Autodesk Fusion 360 part; units mm, degrees
sketch "Sketch1" plane through (0, 0, 0) normal (0, 1, 0) x (1, 0, 0)
  line L0 (0, 0) -> (20, 0)
  line L1 (20, 0) -> (20, 13)
  line L2 (20, 13) -> (0, 13)
  line L3 (0, 3) -> (11, 3)
  line L4 (11, 3) -> (11, 10)
  line L5 (11, 10) -> (0, 10)
  line L6 (0, 13) -> (0, 10)
  line L7 (0, 3) -> (0, 0)
  circle A0 centre (15.5354, 6.5333) radius 3
  dimension "d2" = 6
sketch "Sketch2" plane through (0, 0, 0) normal (0, 1, 0) x (-1, 0, 0)
  line L0 (0, -3) -> (-11, -3)
  line L1 (-20, -13) -> (0, -13)
  circle A0 centre (-15.5354, -6.5333) radius 3
  dimension "d3" = 11
  dimension "d4" = 20
  dimension "d5" = 6
extrude "Extrude1" add sketch "Sketch2" against normal blind 22
extrude "Extrude2" add sketch "Sketch1" against normal blind 2
sketch "Sketch3" plane through (20, 0, 0) normal (1, 0, 0) x (0, 1, 0)
  line L0 (0, -13) -> (0, 0)
  line L1 (0, 0) -> (-2, 0)
  line L2 (-2, 0) -> (-2, -13)
  line L3 (-2, -13) -> (0, -13)
extrude "Extrude3" add 1 faces at (15.9008, -22, -5.6024) along direction (0, -1, 0) blind 10
Can you work these out from the model? Positions are in its coordinate system, mm. A direction names the side the tool comes from. Coordinates: 2 decimals unless noted, no trailing zeros. Loops run counter-clockwise (first coordinate to the right, second up) from the corner with the lowest first, then second, coordinate; pieces in that order, holes last. Notation, with made-up numbers: (-13.5, 30) -> (4.5, 30) arc R30 cw to (4.5, 69) -> close; hole circle Ø10 at (11.25, 20.5). An arc over 180 degrees is marked (long way). Answer as a JSON object with one key per item and string values.
1) Thinking about a two-plate mould opening in Z: for faces 1 (the face through (20, -1, -6)), 2 (the face through (11, -1, -6)), 3 (the face through (5, -1, -3)), 4 (the face through (10, -1, -13)), which applies, pulls with the +Z half, pulls with the -Z half, needs draft (parallel to the pull), parting line crosses it, or undercut?
Results:
{"face 1": "needs draft", "face 2": "undercut", "face 3": "undercut", "face 4": "pulls with the -Z half"}
2) For P1, Ø5, axis at y = -14.5, z = -8.5, coming from the -X side; P2, Ø4, axis at y = -24, z = -8, coming from the +X side; P3, Ø6, axis at x = 13, y = -18.5, coming from the +Z side; P4, Ø0.6, axis at x = 8, y = -1.5, coming from the +Z side, each with a flat end and sliding along its axis, tell me the tip position at first contact or that it passes through.
Results:
{"P1": "stops at x = 12.54", "P2": "stops at x = 18.54", "P3": "stops at z = -3.53", "P4": "stops at z = 0"}
3) Imagine slicing it at B-B (z = -6). Please give me the cut outline in (x, y).
Results:
{"outline": "(11, -2) -> (12.58, -2) -> (12.58, -32) -> (18.49, -32) -> (18.49, -2) -> (20, -2) -> (20, 0) -> (11, 0) -> close"}
4) If I drill on line 1 (Y direction, x = 18, z = -0.5); line 2 (X direction, y = -22.5, z = -7.25); line 3 (X direction, y = -3, z = -7), over which ranges is the centre line in solid material (lowest first)?
Results:
{"line 1": "y = -2 to 0", "line 2": "x = 12.62 to 18.45", "line 3": "x = 12.57 to 18.5"}
5) For faces 5 (the face through (6, -1, -10)), 6 (the face through (17.916, -16.79, -8.359)), 7 (the face through (12, 0, -7)), which set-ups out of +Z, -Z, +X, -X, +Y, -Y let a thin tool reach every point of the face, with its end or its side?
Results:
{"face 5": "-X, +Y, -Y", "face 6": "-Y", "face 7": "+Z, -Z, +X, -X, +Y"}
6) Imagine slicing it at A-A (x = 3.75). Please give me the cut outline in (y, z), then the cut area to 3 significant figures.
Results:
{"outline": "(-2, -13) -> (0, -13) -> (0, -10) -> (-2, -10) -> close; (-2, -3) -> (0, -3) -> (0, 0) -> (-2, 0) -> close", "area": "12.0 mm^2"}
7) Imagine slicing it at D-D (z = -1). Please give me the cut outline in (x, y).
Results:
{"outline": "(0, -2) -> (20, -2) -> (20, 0) -> (0, 0) -> close"}
8) Imagine slicing it at C-C (y = -1.5). Please give me the cut outline in (x, z).
Results:
{"outline": "(0, -13) -> (20, -13) -> (20, 0) -> (0, 0) -> (0, -3) -> (11, -3) -> (11, -10) -> (0, -10) -> close"}
